Source: CAD feature listing. Evaluate the final solid. Frame: model axes, mm. Give positions to 0.01 mm unless a question says otherwise; leave off trailing zeros. Order: outer loops, then holes, each group sorted by start corner. A loop starts at its lowest first (then second) coordinate and runs counter-clockwise, first axis right, second up. Notation, with made-up numbers: (-16.75, -16.5) - (34.25, -16.5) arc R23 ccw to (34.25, -1.5) - close; hole circle Ø5 at (-15.5, 42). An arc over 180 degrees is marked (long way). Write each question's results on one line, items separated by ' | '. Start each with the question number.
Item 1: Section B-B on x = 0. Output: boundary loops of the cut face in (y, z).
Item 2: Mould query, pull axis X, two halves, no side actions, for faces 1 (the cylindrical face through (14.207, 26.433, 2.465)), 2 (the flat face through (0, 32.5, 2)), 3 (the cylindrical face through (-18.43, 31.98, 2.54)). Classes: released by +X, released by -X, zero draft, split by the parting line, or undercut.
Item 3: Section D-D on y = -8. Output: boundary loops of the cut face in (x, z), and give its area (3 significant figures).
Item 4: Line query: line 1 along Y through (x, z) = (-14.5, 3.1); line 2 along Y through (x, z) = (0, 1.1); line 3 along X through (y, z) = (24, 0.4). Output: solid intervals per line, ascending.
Item 5: Section C-C on z = 1.7. Output: boundary loops of the cut face in (x, y), and give its area (3 significant figures).
Item 6: Contact query for flat-ended pins moving along their axis: pin 1 Ø3 at (x, z) = (26, 2) entering from -Y; pin 2 Ø1.5 at (y, z) = (8.5, 3.5) entering from +X; pin 3 Ø1.5 at (y, z) = (24, 4) entering from +X. Output: stop coordinate, or through.
Item 7: Section A-A on x = -14.5. Output: boundary loops of the cut face in (y, z).
Autodesk Inventor part; units mm, degrees
ref_plane "YZ Plane" through (0, 0, 0) normal (1, 0, 0) x (0, 1, 0)
ref_plane "XZ Plane" through (0, 0, 0) normal (0, 1, 0) x (-1, 0, 0)
ref_plane "XY Plane" through (0, 0, 0) normal (0, 0, 1) x (1, 0, 0)
sketch "Sketch1" plane through (0, 0, 0) normal (0, 0, 1) x (1, 0, 0)
  line L0 (-14.5, 25.1147) -> (14.5, 25.1147) construction
  line L1 (14.5, 25.1147) -> (29, 0) construction
  line L2 (29, 0) -> (14.5, -25.1147) construction
  line L3 (14.5, -25.1147) -> (-14.5, -25.1147) construction
  line L4 (-14.5, -25.1147) -> (-29, 0) construction
  line L5 (-29, 0) -> (-14.5, 25.1147) construction
  line L6 (-18.7639, 32.5) -> (18.7639, 32.5)
  line L7 (18.7639, 32.5) -> (37.5278, 0)
  line L8 (37.5278, 0) -> (18.7639, -32.5)
  line L9 (18.7639, -32.5) -> (-18.7639, -32.5)
  line L10 (-18.7639, -32.5) -> (-37.5278, 0)
  line L11 (-37.5278, 0) -> (-18.7639, 32.5)
  circle A0 centre (-14.5, 25.1147) radius 11 construction
  circle A1 centre (14.5, 25.1147) radius 11 construction
  circle A2 centre (29, 0) radius 11 construction
  circle A3 centre (14.5, -25.1147) radius 11 construction
  circle A4 centre (-14.5, -25.1147) radius 11 construction
  circle A5 centre (-29, 0) radius 11 construction
  circle A6 centre (-14.5, 25.1147) radius 1.35
  circle A7 centre (14.5, 25.1147) radius 1.35
  circle A8 centre (29, 0) radius 1.35
  circle A9 centre (14.5, -25.1147) radius 1.35
  circle A10 centre (-14.5, -25.1147) radius 1.35
  circle A11 centre (-29, 0) radius 1.35
  circle A12 centre (0, 0) radius 4
  circle A13 centre (0, 0) radius 40 construction
  dimension "d0" = 22
  dimension "d1" = 50.2295
  dimension "d2" = 2.7
  dimension "d3" = 65
  dimension "d4" = 8
  dimension "d8" = 80
extrude "Extrusion1" add sketch "Sketch1" along normal blind 5
fillet "Fillet1" radius 4 6 edges at (37.5278, 0, 2.5) (18.7639, -32.5, 2.5) (-18.7639, -32.5, 2.5) (-37.5278, 0, 2.5) (-18.7639, 32.5, 2.5) (18.7639, 32.5, 2.5)
properties part number "rotor 1"
Evaluation:
1) outline: (-32.5, 0) - (-4, 0) - (-4, 5) - (-32.5, 5) - close; (4, 0) - (32.5, 0) - (32.5, 5) - (4, 5) - close
2) face 1: undercut | face 2: zero draft | face 3: released by -X
3) outline: (-32.91, 0) - (32.91, 0) - (32.91, 5) - (-32.91, 5) - close | area: 329 mm^2
4) line 1: y = -32.5 to -26.46, -23.76 to 23.76, 26.46 to 32.5 | line 2: y = -32.5 to -4, 4 to 32.5 | line 3: x = -23.67 to -15.26, -13.74 to 13.74, 15.26 to 23.67
5) outline: (-36.37, -2) - (-19.92, -30.5) arc R4 ccw to (-16.45, -32.5) - (16.45, -32.5) arc R4 ccw to (19.92, -30.5) - (36.37, -2) arc R4 ccw to (36.37, 2) - (19.92, 30.5) arc R4 ccw to (16.45, 32.5) - (-16.45, 32.5) arc R4 ccw to (-19.92, 30.5) - (-36.37, 2) arc R4 ccw to start; hole circle Ø2.7 at (-29, 0); hole circle Ø2.7 at (-14.5, -25.11); hole circle Ø2.7 at (-14.5, 25.11); hole circle Ø8 at (0, 0); hole circle Ø2.7 at (14.5, -25.11); hole circle Ø2.7 at (14.5, 25.11); hole circle Ø2.7 at (29, 0) | area: 3,570 mm^2
6) pin 1: stops at y = -22.56 | pin 2: stops at x = 33.05 | pin 3: stops at x = 24.1
7) outline: (-32.5, 0) - (-26.46, 0) - (-26.46, 5) - (-32.5, 5) - close; (-23.76, 0) - (23.76, 0) - (23.76, 5) - (-23.76, 5) - close; (26.46, 0) - (32.5, 0) - (32.5, 5) - (26.46, 5) - close
